Drawing for the job (mm, zero at the part's lowest x, y, z). A direction names the side the tool comes from. Give positions to 0.01 mm unless a question says otherwise; leave off trailing zeros. Order: outer loops, then holes, each group sorted by start corner. A loop starts at its lowest first (then second) coordinate and runs counter-clockwise, first axis right, second up. Notation, with made-up numbers: (-10, -24.75) - (11, -24.75) arc R24 ccw to (11, 6.25) - close; hole circle Ø9 at (-17, 4.25). An arc over 180 degrees is marked (long way). Use a Markdown table: item, result. Add a question column.
(1) Slice it at D-D (z = 8). Write the cut outline in (x, y), then the cut area to 3 significant figures.
(2) Which spindle directions (+Z, -Z, +X, -X, +Y, -Y) get a long thin tool onto all of the face, cutting with end or side? Do the marked faces 1, 2, 3 and 4. Say none if no direction does.
(3) Wall check: line 1 (Z direction, x = 5.5, y = 12.75); line 2 (Z direction, x = 13.5, y = 2); line 3 (Y direction, x = 18.5, z = 9.5). Give the ranges that are in metal, low to high.
(4) Flat gauge pins, fed straight in: pin 1 (5 mm diameter, centred on x = 16.5, z = 6, fed in from -Y); pin 2 (4 mm diameter, centred on y = 17, z = 10, fed in from -X); pin 3 (7 mm diameter, centred on x = 10.5, z = 10, fed in from +Y); pin 4 (11 mm diameter, centred on y = 18.5, z = 9.5, fed in from +X). Where does each tip first touch, or does it go through?
(5) Mould opens along Y. For the marked faces 5, 6 and 7 say: +Y half, -Y half, draft (parallel to the pull), parting line (faces both ways), or undercut.
(6) Slice it at B-B (x = 17). Write the cut outline in (y, z).
(7) Slice it at A-A (y = 4.5). Write the cut outline in (x, z).
(8) Slice it at C-C (z = 16). Write the cut outline in (x, y), then the cut area to 3 significant figures.
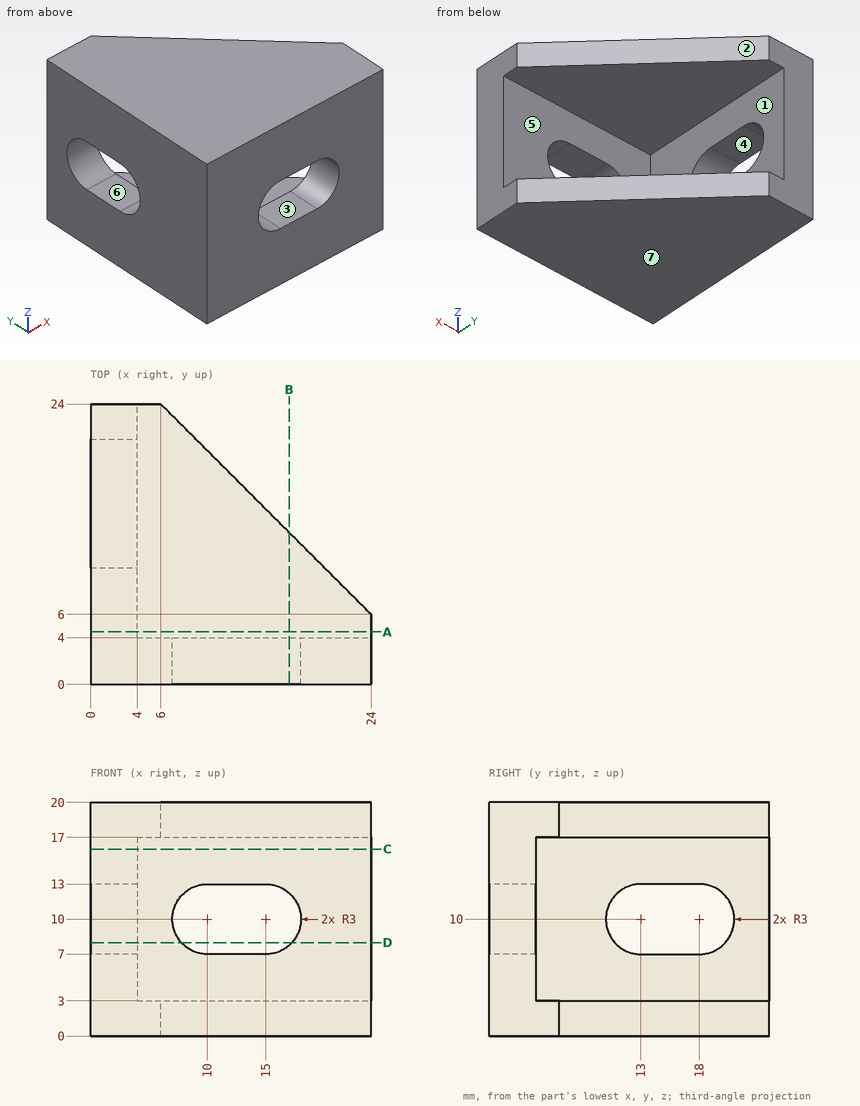
Solution:
| question | item | result |
|---|---|---|
| 1 | outline | (0, 0) - (7.76, 0) - (7.76, 4) - (4, 4) - (4, 10.76) - (0, 10.76) - close; (0, 20.24) - (4, 20.24) - (4, 24) - (0, 24) - close; (17.24, 0) - (24, 0) - (24, 4) - (17.24, 4) - close |
| 1 | area | 100 mm2 |
| 2 | face 1 | +X, +Y |
| 2 | face 2 | +Z, -Z, +X, +Y |
| 2 | face 3 | +Y, -Y |
| 2 | face 4 | +X, -X |
| 3 | line 1 | 0 to 3, 17 to 20 |
| 3 | line 2 | 0 to 7, 13 to 20 |
| 3 | line 3 | 0 to 4 |
| 4 | pin 1 | y = 0 |
| 4 | pin 2 | through |
| 4 | pin 3 | y = 4 |
| 4 | pin 4 | x = 4 |
| 5 | face 5 | +Y half |
| 5 | face 6 | undercut |
| 5 | face 7 | draft |
| 6 | outline | (0, 0) - (13, 0) - (13, 3) - (4, 3) - (4, 7.76) - (0, 7.76) - close; (0, 12.24) - (4, 12.24) - (4, 17) - (13, 17) - (13, 20) - (0, 20) - close |
| 7 | outline | (0, 0) - (24, 0) - (24, 3) - (4, 3) - (4, 17) - (24, 17) - (24, 20) - (0, 20) - close |
| 8 | outline | (0, 0) - (24, 0) - (24, 4) - (4, 4) - (4, 24) - (0, 24) - close |
| 8 | area | 176 mm2 |
